from build123d import *

# Parameters (mm, degrees)
F1_DEPTH = 12.7


with BuildPart() as f1:
    # F0 (on Front) → F1 (new body)
    with BuildSketch(Plane.XZ):
        Polygon((-33.7118367519, 41.1562249064), (-40.6031636763, 33.6906229065), (-6.4398701091, 0.0998017263), (0.842697291, 7.1807192451), align=None)
        Polygon((0.842697291, 7.1807192451), (-6.4398701091, 0.0998017263), (-2.4844633379, -3.7893245163), (0.0352224959, -6.2667881165), (7.317789896, 0.8141294024), align=None)
        Polygon((-2.4844633379, -3.7893245163), (-6.4398701091, 0.0998017263), (-40.6031636763, -33.1175309299), (-33.4843747504, -40.357643914), (0.0352224959, -6.2667881165), align=None)
        Polygon((34.2488773167, 41.1562249064), (0.842697291, 7.1807192451), (7.317789896, 0.8141294024), (40.9988134673, 33.5625458269), align=None)
        Polygon((40.9988134673, -32.3025031532), (7.317789896, 0.8141294024), (0.0352224959, -6.2667881165), (33.1869239615, -39.9834872244), align=None)
    extrude(amount=F1_DEPTH)


solid = f1.part
The model under review builds one solid part; all positions refer to its coordinate system, in mm. A direction names the side the tool comes from. Coordinates: 2 decimals unless noted, no trailing zeros. Write each loop counter-clockwise with the first axis right and the second up, starting at its lowest first coordinate (ties: lowest second). Pieces come first, ordered by that corner, then holes. Notation, with made-up numbers: M 76.25,71 L 93.25,71 A24 cw 93.25,94 Z; hole C 55.5,-37 d3. An arc over 180 degrees is marked long. Put each result on its own line as item: value.
1) Add section B-B on z = -25.5. Give the boundary of the cut face in (x, y), then the cut area to 3 significant figures.
Computed:
outline: M -32.77,-12.7 L -18.88,-12.7 L -18.88,0 L -32.77,0 Z; M 18.95,-12.7 L 34.08,-12.7 L 34.08,0 L 18.95,0 Z
area: 369 mm2
2) Clearance check with flat-ended pins moving along their axes: pin 1 Ø3 at (x, y) = (-9, -7.5) entering from -Z; pin 2 Ø2 at (x, y) = (20.5, -11) entering from -Z; pin 3 Ø2 at (x, y) = (-11, -6) entering from +Z. State where each tip first meets the part, or that it passes through.
Computed:
pin 1: stops at z = -16.98
pin 2: stops at z = -28.1
pin 3: stops at z = 19.81
3) Draft analysis for pull direction Z (two halves, no side actions). For faces 5 (the flat face through (-3, -12.7, 1)), 6 (the flat face through (37.038, -6.261, -36.197)), 7 (the flat face through (24.394, -6.261, -15.976)), 8 (the flat face through (-16.19, -6.26, 23.93)), state which applies: released by +Z, released by -Z, zero draft, split by the parting line, or undercut.
Computed:
face 5: zero draft
face 6: released by -Z
face 7: undercut
face 8: released by +Z
4) Add section D-D on x = -5. Give the boundary of the cut face in (y, z).
Computed:
outline: M -12.7,-11.39 L 0,-11.39 L 0,12.93 L -12.7,12.93 Z
5) For faces 1 (the flat face through (-23, -6, -16)), 2 (the flat face through (23.923, -6.261, 16.959)), 3 (the flat face through (17.78, -6.261, 24.406)), 4 (the flat face through (-16.96, -6.26, -23.55)), list the 3-axis set-ups (+Z, -Z, +X, -X, +Y, -Y) from which the entire face can be reached by the end or side of a thin tool; tool diameter is ignored.
Computed:
face 1: -X, +Y, -Y
face 2: +X, +Y, -Y
face 3: +Z, +Y, -Y
face 4: -Z, +Y, -Y
6) Wall thickness on probe 1 along X at (y, z) = (-5.75, 36.5); probe 2 along X at (y, z) = (-9.5, -22); probe 3 along Z at (x, y) = (-35, -9.25): over which ranges is each line inside the solid? List them lowest first. Write a range as [from, to].
Computed:
probe 1: x = [-38.01, -28.98], [29.67, 38.39]
probe 2: x = [-29.17, -15.43], [15.5, 30.52]
probe 3: z = [-38.82, -27.67], [28.18, 39.76]
7) Add section C-C on y = -10.25. Give the boundary of the cut face in (x, z).
Computed:
outline: M -40.6,-33.12 L -33.48,-40.36 L 0.04,-6.27 L 33.19,-39.98 L 41,-32.3 L 7.32,0.81 L 41,33.56 L 34.25,41.16 L 0.84,7.18 L -33.71,41.16 L -40.6,33.69 L -6.44,0.1 Z
8) Add section A-A on x = 17. Give the boundary of the cut face in (y, z).
Computed:
outline: M -12.7,-23.52 L 0,-23.52 L 0,-8.71 L -12.7,-8.71 Z; M -12.7,10.23 L 0,10.23 L 0,23.61 L -12.7,23.61 Z
